The drawing under review shows one solid part. Ordinate dimensions are in mm from its lowest x, y, z. Coordinates: 2 decimals unless noted, no trailing zeros. Loops run counter-clockwise (first coordinate to the right, second up) from the corner with the lowest first, then second, coordinate; pieces in that order, holes last. Notation, with made-up numbers: (83, 58.5) -> (130, 58.5) arc R19 ccw to (130, 81.5) -> close; hole circle Ø3 at (-21.75, 74.25). An arc over 180 degrees is marked (long way). Use a Markdown table: item, result.
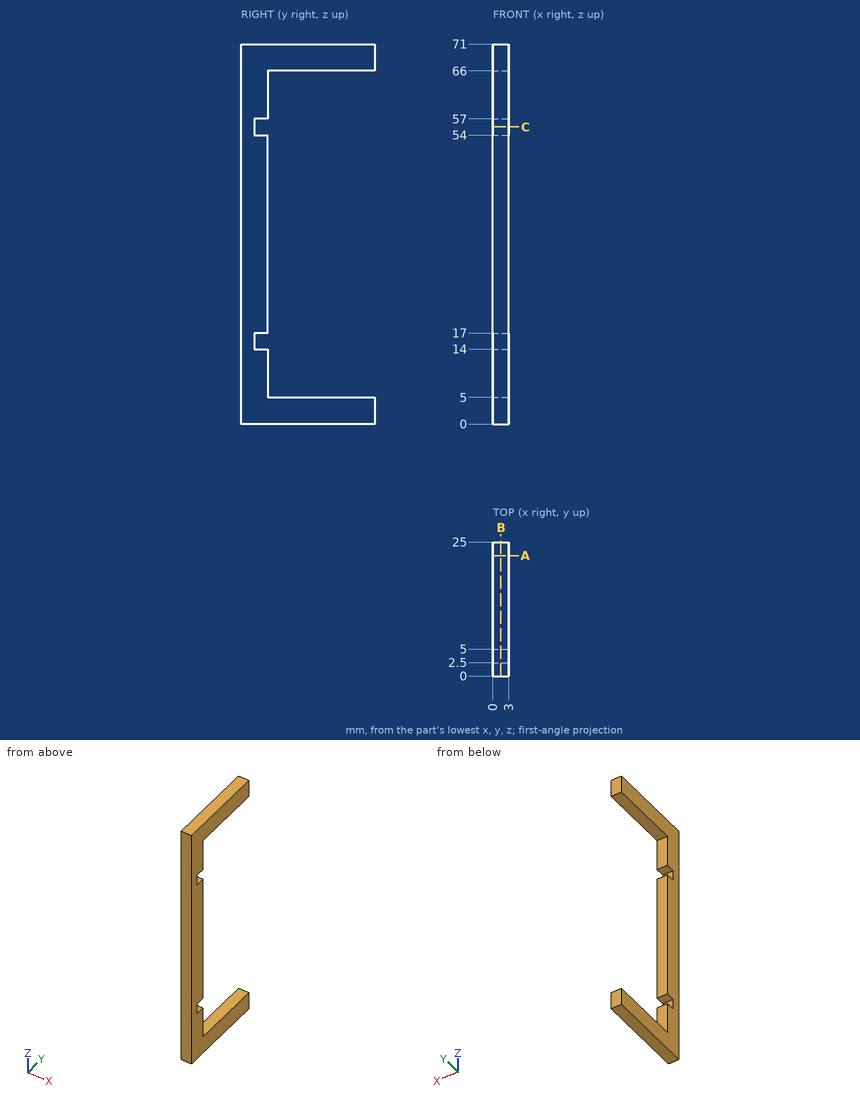
(1) Take a section at A-A on y = 22.5. Write out the cut boundary in (x, z).
Found:
| item | result |
|---|---|
| outline | (0, 0) -> (3, 0) -> (3, 5) -> (0, 5) -> close; (0, 66) -> (3, 66) -> (3, 71) -> (0, 71) -> close |
(2) For pin 1 Ø0.9 at (x, z) = (1, 11) entering from +Y; pin 2 Ø0.9 at (x, z) = (1.5, 15.5) entering from +Y, all flat-tipped, find the tip position at first contact; note any pin that passes through.
Found:
| item | result |
|---|---|
| pin 1 | stops at y = 5 |
| pin 2 | stops at y = 2.5 |
(3) For line 1 along Z through (x, y) = (2.2, 3.25); line 2 along Z through (x, y) = (1.85, 21); line 3 along Y through (x, z) = (2.5, 16.5), list the stretches that pass through material, from the lowest coordinate up.
Found:
| item | result |
|---|---|
| line 1 | z = 0 to 14, 17 to 54, 57 to 71 |
| line 2 | z = 0 to 5, 66 to 71 |
| line 3 | y = 0 to 2.5 |
(4) Take a section at B-B on x = 1.5. Write out the cut boundary in (y, z), plus the area to 3 significant figures.
Found:
| item | result |
|---|---|
| outline | (0, 0) -> (25, 0) -> (25, 5) -> (5, 5) -> (5, 14) -> (2.5, 14) -> (2.5, 17) -> (5, 17) -> (5, 54) -> (2.5, 54) -> (2.5, 57) -> (5, 57) -> (5, 66) -> (25, 66) -> (25, 71) -> (0, 71) -> close |
| area | 540 mm^2 |
(5) Take a section at C-C on z = 55.5. Write out the cut boundary in (x, y).
Found:
| item | result |
|---|---|
| outline | (0, 0) -> (3, 0) -> (3, 2.5) -> (0, 2.5) -> close |
